Autodesk Inventor part; units mm, degrees
ref_plane "YZ Plane" through (0, 0, 0) normal (1, 0, 0) x (0, 1, 0)
ref_plane "XZ Plane" through (0, 0, 0) normal (0, 1, 0) x (-1, 0, 0)
ref_plane "XY Plane" through (0, 0, 0) normal (0, 0, 1) x (1, 0, 0)
sketch "스케치1" plane through (0, 0, 0) normal (0, 0, 1) x (1, 0, 0)
  line L0 (-36.25, -33.9) -> (36.25, -33.9)
  line L1 (36.25, -33.9) -> (36.25, 33.9)
  line L2 (36.25, 33.9) -> (-36.25, 33.9)
  line L3 (-36.25, 33.9) -> (-36.25, -33.9)
  line L4 (-36.25, -33.9) -> (36.25, 33.9) construction
  line L5 (36.25, -33.9) -> (-36.25, 33.9) construction
  line L6 (-32.5, -30) -> (32.5, -30) construction
  line L7 (32.5, -30) -> (32.5, 30) construction
  line L8 (32.5, 30) -> (-32.5, 30) construction
  line L9 (-32.5, 30) -> (-32.5, -30) construction
  line L10 (-32.5, -30) -> (32.5, 30) construction
  line L11 (32.5, -30) -> (-32.5, 30) construction
  circle A0 centre (-32.5, 30) radius 1.75
  circle A1 centre (-32.5, -30) radius 1.75
  line L12 (0, 0) -> (0, 9.9513)
  circle A2 centre (32.5, 30) radius 1.75
  circle A3 centre (32.5, -30) radius 1.75
  dimension "d0" = 72.5
  dimension "d1" = 67.8
  dimension "d2" = 65
  dimension "d3" = 60
  dimension "d4" = 3.5
  dimension "d5" = 3.5
extrude "돌출1" add sketch "스케치1" along normal blind 1.55
sketch "스케치2" plane through (0, 0, 1.55) normal (0, 0, 1) x (1, 0, 0)
  circle A0 centre (32.5, -30) radius 1.75
  circle A1 centre (-32.5, -30) radius 1.75
  circle A2 centre (-32.5, 30) radius 1.75
  line L0 (-36.25, -33.9) -> (36.25, -33.9)
  line L1 (36.25, -33.9) -> (36.25, 33.9)
  line L2 (36.25, 33.9) -> (-36.25, 33.9)
  line L3 (-15.25, -18.9) -> (14.75, -18.9)
  line L4 (14.75, -18.9) -> (14.75, -27.4)
  line L5 (14.75, -27.4) -> (-15.25, -27.4)
  line L6 (-15.25, -27.4) -> (-15.25, -18.9)
  line L7 (-27.25, 0.9) -> (-17.75, 0.9)
  line L8 (-17.75, 0.9) -> (-17.75, -8.1)
  line L9 (-17.75, -8.1) -> (-27.25, -8.1)
  line L10 (-27.25, -8.1) -> (-27.25, 0.9)
  line L11 (-12.25, 0.9) -> (-2.75, 0.9)
  line L12 (-2.75, 0.9) -> (-2.75, -8.1)
  line L13 (-2.75, -8.1) -> (-12.25, -8.1)
  line L14 (-12.25, -8.1) -> (-12.25, 0.9)
  line L15 (3.25, 18.9) -> (16.25, 18.9)
  line L16 (16.25, 18.9) -> (16.25, 10.9)
  line L17 (16.25, 10.9) -> (3.25, 10.9)
  line L18 (3.25, 10.9) -> (3.25, 18.9)
  circle A3 centre (-22.25, -26.4) radius 5
  line L19 (-8.75, 18.9) -> (0.25, 18.9)
  line L20 (0.25, 18.9) -> (0.25, 14.4)
  line L21 (0.25, 14.4) -> (-8.75, 14.4)
  line L22 (-8.75, 14.4) -> (-8.75, 18.9)
  line L23 (15.25, 29.4) -> (23.75, 29.4)
  line L24 (23.75, 29.4) -> (23.75, 24.4)
  line L25 (23.75, 24.4) -> (15.25, 24.4)
  line L26 (15.25, 24.4) -> (15.25, 29.4)
  point P0 (0, 0)
  dimension "d8" = 10
  dimension "d9" = 8.5
  dimension "d10" = 30
  dimension "d11" = 9
  dimension "d12" = 9.5
  dimension "d13" = 9.5
  dimension "d14" = 13
  dimension "d15" = 8
  dimension "d20" = 6.5
  dimension "d21" = 21.5
  dimension "d23" = 5.5
  dimension "d24" = 33
  dimension "d25" = 10
  dimension "d26" = 20
  dimension "d27" = 9
  dimension "d28" = 4.5
  dimension "d29" = 3
  dimension "d30" = 15
  dimension "d32" = 8.5
  dimension "d33" = 5
  dimension "d34" = 12.5
  dimension "d35" = 4.5
  dimension "d36" = 2.5
  dimension "d38" = 65
  dimension "d39" = 60
extrude "돌출2" add sketch "스케치2" along normal blind 12.2 contours A3
extrude "돌출3" add sketch "스케치2" along normal blind 4.5 contours L7 L8 L9 L10 | L11 L12 L13 L14
extrude "돌출4" add sketch "스케치2" along normal blind 10.2 contours L3 L4 L5 L6
extrude "돌출5" add sketch "스케치2" along normal blind 2.5 contours L15 L16 L17 L18
extrude "돌출6" add sketch "스케치2" along normal blind 1.5 contours L19 L20 L21 L22
extrude "돌출7" add sketch "스케치2" along normal blind 8 contours L23 L24 L25 L26
mirror "미러1" about plane through (0, 0, 0) normal (1, 0, 0) of "돌출3"
sketch "스케치4" plane through (0, 0, 0) normal (0, 0, -1) x (-1, 0, 0)
  line L0 (-36.25, -33.9) -> (-36.25, 33.9)
  line L1 (-29.75, 23.1) -> (-29.75, -6.9)
  line L2 (-29.75, -6.9) -> (29.75, -6.9)
  line L3 (29.75, -6.9) -> (29.75, 23.1)
  line L4 (29.75, 23.1) -> (-29.75, 23.1)
  line L5 (36.25, -33.9) -> (-36.25, -33.9)
  point P0 (0, 0)
  point P1 (0, 23.1)
  point P2 (-36.25, 0)
  dimension "d53" = 59.5
  dimension "d54" = 30
  dimension "d58" = 27
extrude "돌출8" add sketch "스케치4" along normal blind 10
properties part number "모터드라이버"
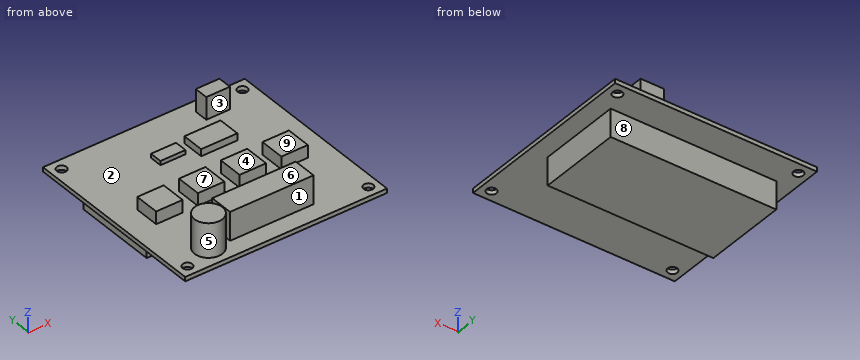
Here's how the part is built. I have some questions about the finished solid (model axes, mm). Face numbers are marked on the shaded views. A direction names the side the tool comes from. Give positions to 0.01 mm unless a question says otherwise; leave off trailing zeros. Order: outer loops, then holes, each group sorted by start corner. A loop starts at its lowest first (then second) coordinate and runs counter-clockwise, first axis right, second up. Notation, with made-up numbers: (-36, -5) -> (-9, -5) arc R9 cw to (-9, 2) -> close; hole circle Ø10 at (40.5, -3). An arc over 180 degrees is marked (long way). One line per item, written item: value. Start each with the question number.
1. Will these pins go through, and if not, where does the flat tip stop? pin 1 Ø2 at (x, z) = (10, 9.5) entering from +Y; pin 2 Ø0.8 at (y, z) = (15, 3) entering from -X; pin 3 Ø2 at (x, z) = (-10, 3) entering from +Y; pin 4 Ø10 at (x, z) = (22, -0.5) entering from +Y.
2. Imagine slicing it at C-C, the plane x = -7.5. List the corners of the cut face in (y, z) for me, plus the area to 3 significant figures.
3. For the marked faces 5, 6, 7, 8 and 9, which set-ups out of +Z, -Z, +X, -X, +Y, -Y let a thin tool reach every point of the face, with its end or its side?
4. Imagine slicing it at A-A, the plane x = 32.5. List the corners of the cut face in (y, z) for me, plus the area to 3 significant figures.
5. Imagine slicing it at D-D, the plane z = -6. List the corners of the cut face in (x, y) for me.
6. We'd pull the mould along Y, two halves only. Please class the marked faces 1, 2, 3 and 4: released by +Y, released by -Y, zero draft, split by the parting line, or undercut.
7. I need wall thicknesses on probe 1 along X at (y, z) = (-2.5, 3.75); probe 2 along Y at (x, z) = (32.5, 0.6); probe 3 along Y at (x, z) = (18.5, -8). Which ranges of each line are inside material? Lowest first, please. Write a range as from..to.
8. Imagine slicing it at B-B, the plane y = -26.4. List the corners of the cut face in (x, z) for me.
Values follow:
1. pin 1: stops at y = -18.9
1. pin 2: stops at x = -8.75
1. pin 3: stops at y = 0.9
1. pin 4: stops at y = 33.9
2. outline: (-33.9, 0) -> (-6.9, 0) -> (-6.9, -10) -> (23.1, -10) -> (23.1, 0) -> (33.9, 0) -> (33.9, 1.55) -> (18.9, 1.55) -> (18.9, 3.05) -> (14.4, 3.05) -> (14.4, 1.55) -> (0.9, 1.55) -> (0.9, 6.05) -> (-8.1, 6.05) -> (-8.1, 1.55) -> (-18.9, 1.55) -> (-18.9, 11.75) -> (-27.4, 11.75) -> (-27.4, 1.55) -> (-33.9, 1.55) -> close
2. area: 539 mm2
3. face 5: +Z
3. face 6: +Z, +X, +Y, -Y
3. face 7: +Z, +X, -X, +Y
3. face 8: -Z, +X, -X, +Y
3. face 9: +Z, +X, -X, -Y
4. outline: (-33.9, 0) -> (-31.75, 0) -> (-31.75, 1.55) -> (-33.9, 1.55) -> close; (-28.25, 0) -> (28.25, 0) -> (28.25, 1.55) -> (-28.25, 1.55) -> close; (31.75, 0) -> (33.9, 0) -> (33.9, 1.55) -> (31.75, 1.55) -> close
4. area: 94.2 mm2
5. outline: (-29.75, -6.9) -> (29.75, -6.9) -> (29.75, 23.1) -> (-29.75, 23.1) -> close
6. face 1: released by -Y
6. face 2: undercut
6. face 3: undercut
6. face 4: zero draft
7. probe 1: x = -27.25..-17.75, -12.25..-2.75, 2.75..12.25, 17.75..27.25
7. probe 2: y = -33.9..-31.75, -28.25..28.25, 31.75..33.9
7. probe 3: y = -6.9..23.1
8. outline: (-36.25, 0) -> (36.25, 0) -> (36.25, 1.55) -> (14.75, 1.55) -> (14.75, 11.75) -> (-15.25, 11.75) -> (-15.25, 1.55) -> (-17.25, 1.55) -> (-17.25, 13.75) -> (-27.25, 13.75) -> (-27.25, 1.55) -> (-36.25, 1.55) -> close
